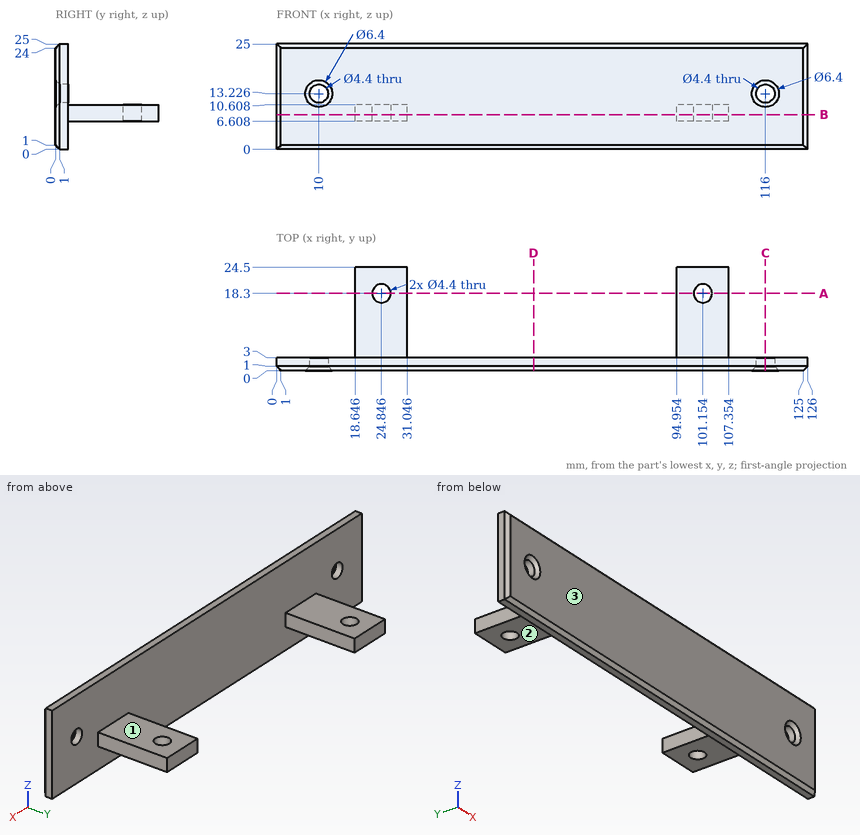
Answer from the drawing. Dimensions are ordinates in mm from the lowest x, y and z of the part. A direction names the side the tool comes from. Give positions to 0.01 mm unless a question says otherwise; leave off trailing zeros. Order: outer loops, then holes, each group sorted by start corner. A loop starts at its lowest first (then second) coordinate and runs counter-clockwise, first axis right, second up. Notation, with made-up numbers: (89.5, 86) -> (115.5, 86) arc R20 ccw to (115.5, 102) -> close; hole circle Ø1 at (5.5, 11.5). An arc over 180 degrees is marked (long way). One line per item, written item: value. Start each with the question number.
(1) The part is cut by section C-C (x = 116). Determine the outline of the cut face in (y, z), and give its area (3 significant figures).
(2) Flat-ended cylindrical pins translate along their axes: P1, Ø6, axis at x = 103, y = 17.5, coming from the -Z side; P2, Ø10, axis at x = 112.5, z = 2.5, coming from the +Y side; P3, Ø3.5, axis at x = 24, y = 18, coming from the +Z side. Find the tip coordinate at first contact, or state that the pin passes through.
(3) Straight lines are drawn through the part: L1, parallel to Z at x = 10, y = 1.65; L2, parallel to Y at x = 87, z = 9.5; L3, parallel to Z at x = 104.5, y = 12.5. For each, find the intervals that lie inside material, in ascending order.
(4) The part is cut by section D-D (x = 61). Determine the outline of the cut face in (y, z), and give its area (3 significant figures).
(5) The part is cut by section A-A (y = 18.3). Determine the outline of the cut face in (x, z).
(6) A tool of negligible diameter and unlimited length cuts with its end or side. For the marked faces 1, 2 and 3, from which of +Z, -Z, +X, -X, +Y, -Y can it reach the whole face along a straight path? Write none if from no direction.
(7) The part is cut by section B-B (z = 8.25). Determine the outline of the cut face in (x, y), and give its area (3 significant figures).
Taken from the geometry:
1. outline: (0, 1) -> (1, 0) -> (3, 0) -> (3, 11.03) -> (1, 11.03) -> (0, 10.03) -> close; (0, 16.43) -> (1, 15.43) -> (3, 15.43) -> (3, 25) -> (1, 25) -> (0, 24) -> close
1. area: 59.8 mm^2
2. P1: z = 6.61
2. P2: y = 3
2. P3: z = 10.61
3. L1: 0 to 11.03, 15.43 to 25
3. L2: 0 to 3
3. L3: 6.61 to 10.61
4. outline: (0, 1) -> (1, 0) -> (3, 0) -> (3, 25) -> (1, 25) -> (0, 24) -> close
4. area: 74.0 mm^2
5. outline: (18.65, 6.61) -> (22.65, 6.61) -> (22.65, 10.61) -> (18.65, 10.61) -> close; (27.05, 6.61) -> (31.05, 6.61) -> (31.05, 10.61) -> (27.05, 10.61) -> close; (94.95, 6.61) -> (98.95, 6.61) -> (98.95, 10.61) -> (94.95, 10.61) -> close; (103.35, 6.61) -> (107.35, 6.61) -> (107.35, 10.61) -> (103.35, 10.61) -> close
6. face 1: +Z, +X, -X, +Y
6. face 2: -Z, +X, -X, +Y
6. face 3: +Z, -Z, +X, -X, -Y
7. outline: (0, 1) -> (1, 0) -> (125, 0) -> (126, 1) -> (126, 3) -> (107.35, 3) -> (107.35, 24.5) -> (94.95, 24.5) -> (94.95, 3) -> (31.05, 3) -> (31.05, 24.5) -> (18.65, 24.5) -> (18.65, 3) -> (0, 3) -> close; hole circle Ø4.4 at (24.85, 18.3); hole circle Ø4.4 at (101.15, 18.3)
7. area: 880 mm^2
